Source: CAD feature listing. Evaluate the final solid. Frame: model axes, mm. Give positions to 0.01 mm unless a question says otherwise; leave off trailing zeros. Write each loop counter-clockwise with the first axis right and the second up, starting at its lowest first coordinate (ties: lowest second). Pieces come first, ordered by that corner, then holes. Notation, with made-up numbers: (89, 0.25) - (112, 0.25) arc R25 ccw to (112, 24.25) - close; hole circle Ø6 at (-12, 16). An arc over 180 degrees is marked (long way). One line per question, with ' | ' between items. Start each with the question number.
(1) Section A-A, the plane z = 0.1. Return loops of the section in (x, y).
(2) Section B-B, the plane x = -51.5. Return loops of the section in (y, z), plus the area to 3 significant figures.
(3) Ray query, line 1 (X direction, y = 5, z = 0.15); line 2 (Y direction, x = -23, z = 0.1). Return the intervals inside material, ascending. Write a range as [from, to].
```python
from build123d import *

# Parameters (mm, degrees)
SKETCH1_W           = 76.2
SKETCH1_H           = 69.85
BOSS_EXTRUDE1_DEPTH = 0.396875
SKETCH2_W           = 5.08
SKETCH2_H           = 5.08
CUT_EXTRUDE1_DEPTH  = 1.396875


with BuildPart() as part:
    # Sketch1 → Boss-Extrude1 (new body)
    with BuildSketch(Plane.XY):
        with Locations((-38.1, 34.925)):
            Rectangle(SKETCH1_W, SKETCH1_H)
    extrude(amount=BOSS_EXTRUDE1_DEPTH)

    # Sketch2 → Cut-Extrude1 (cut, through all)
    with BuildSketch(Plane(origin=(0, 0, 0), x_dir=(-1, 0, 0), z_dir=(0, 0, -1))):
        with Locations((63.5, 5.08)):
            Rectangle(SKETCH2_W, SKETCH2_H)
        with Locations((50.8, 5.08)):
            Rectangle(SKETCH2_W, SKETCH2_H)
        with Locations((38.1, 5.08)):
            Rectangle(SKETCH2_W, SKETCH2_H)
        with Locations((25.4, 5.08)):
            Rectangle(SKETCH2_W, SKETCH2_H)
        with Locations((12.7, 5.08)):
            Rectangle(SKETCH2_W, SKETCH2_H)
    extrude(amount=-CUT_EXTRUDE1_DEPTH, mode=Mode.SUBTRACT)


solid = part.part
```
Check sheet entries:
1) outline: (-76.2, 0) - (0, 0) - (0, 69.85) - (-76.2, 69.85) - close; hole (-66.04, 2.54) - (-60.96, 2.54) - (-60.96, 7.62) - (-66.04, 7.62) - close; hole (-53.34, 2.54) - (-48.26, 2.54) - (-48.26, 7.62) - (-53.34, 7.62) - close; hole (-40.64, 2.54) - (-35.56, 2.54) - (-35.56, 7.62) - (-40.64, 7.62) - close; hole (-27.94, 2.54) - (-22.86, 2.54) - (-22.86, 7.62) - (-27.94, 7.62) - close; hole (-15.24, 2.54) - (-10.16, 2.54) - (-10.16, 7.62) - (-15.24, 7.62) - close
2) outline: (0, 0) - (2.54, 0) - (2.54, 0.4) - (0, 0.4) - close; (7.62, 0) - (69.85, 0) - (69.85, 0.4) - (7.62, 0.4) - close | area: 25.7 mm²
3) line 1: [-76.2, -66.04], [-60.96, -53.34], [-48.26, -40.64], [-35.56, -27.94], [-22.86, -15.24], [-10.16, 0] | line 2: [0, 2.54], [7.62, 69.85]
